Can you work these out from the model? Positions are in its coordinate system, mm. A direction names the side the tool comes from. Give positions to 0.01 mm unless a question says otherwise; leave off trailing zeros. Write each loop counter-clockwise with the first axis right and the second up, starting at its lowest first coordinate (ties: lowest second). Pieces come first, ordered by that corner, then holes. Notation, with made-up numbers: (68, 13.5) - (96, 13.5) arc R17 cw to (96, 21.5) - close; hole circle Ø4 at (-23.75, 30.25). An arc over 180 degrees is marked (long way). Use a Markdown table: item, result. Add a question column.
Autodesk Fusion 360 part; units mm, degrees
sketch "Sketch1" plane through (0, 0, 0) normal (0, 0, 1) x (1, 0, 0)
  line L0 (0, 0) -> (35, 0)
  line L1 (35, 30) -> (0, 30)
  line L2 (0, 30) -> (0, 0)
  circle A0 centre (35, 15) radius 2.25
  arc A1 (35, 0) -> (35, 30) centre (35, 15) ccw
  line L3 (15, 0) -> (15, 30)
  line L4 (15, 15) -> (0, 30) construction
  line L5 (7.5, 22.5) -> (7.5, 30) construction
  line L6 (7.5, 22.5) -> (0, 22.5) construction
  circle A2 centre (6.5, 23.5) radius 1
  circle A3 centre (8.5, 23.5) radius 1 construction
  circle A4 centre (8.5, 6.5) radius 1
  line L7 (15, 0) -> (0, 15) construction
  line L8 (7.5, 7.5) -> (7.5, 0) construction
  line L9 (7.5, 7.5) -> (15, 7.5) construction
  point P0 (40, 0)
  point P1 (15, 15)
  dimension "d1" = 30
  dimension "d7" = 35
  dimension "d8" = 35
  dimension "d9" = 4.5
  dimension "d14" = 2
  dimension "d36" = 2
extrude "Extrude1" add sketch "Sketch1" along normal blind 5 contours L0 L1 L2 L3 | L0 L1 A1 L3 | A0 | A2 | A4 makes body 1
hole "Hole1" at (8.5, 6.5, 0) at (6.5, 23.5, 0) direction (0, 0, 1) diameter 2 end through all counterbore diameter 2.3 counterbore depth 1 bodies 1 1
sketch "Sketch2" plane through (0, 0, 5) normal (0, 0, 1) x (-1, 0, 0)
  circle A0 centre (-8.5, -6.5) radius 1
  circle A1 centre (-6.5, -23.5) radius 1
  arc A2 (-35, 0) -> (-35, -30) centre (-35, -15) ccw
  line L0 (-35, -30) -> (0, -30)
  line L1 (0, -30) -> (0, 0)
  line L2 (0, 0) -> (-35, 0)
  circle A3 centre (-35, -15) radius 2.25
fillet "Fillet1" radius 2 3 edges at (17.5, 0, 0) (50, 15, 0) (17.5, 30, 0) on bodies 1
ref_plane "WorkPlane1" through (25, 15, 22.5) normal (0, 0, 1) x (1, 0, 0)
mirror "Mirror1" about plane through (25, 15, 22.5) normal (0, 0, 1) of bodies 1 makes body 2
extrude "Extrude2" cut sketch "Sketch2" against normal blind 4 contours A3 bodies 1
sketch "Sketch3" plane through (0, 0, 40) normal (0, 0, -1) x (1, 0, 0)
  circle A0 centre (8.5, -6.5) radius 1
  circle A1 centre (6.5, -23.5) radius 1
  arc A2 (35, -30) -> (35, 0) centre (35, -15) ccw
  line L0 (35, 0) -> (0, 0)
  line L1 (0, 0) -> (0, -30)
  line L2 (0, -30) -> (35, -30)
  line L3 (31.4, -14.9863) -> (24.6174, -26.7346)
  line L4 (35, -15) -> (24.8695, -28.0239) construction
  arc A3 (24.6174, -26.7346) -> (26.1812, -27.951) centre (25.4835, -27.2346) ccw
  line L5 (35.8992, -18.4859) -> (26.1812, -27.951)
  line L6 (31.4, -14.9863) -> (35.8992, -18.4859) construction
  arc A4 (35.8992, -18.4859) -> (31.4, -14.9863) centre (35, -15) ccw
  point P0 (35, -15)
  point P1 (35, -15)
  dimension "d30" = 2
  dimension "d31" = 5.7
  dimension "d32" = 16.5
  dimension "d33" = 7.2
extrude "Extrude3" cut sketch "Sketch3" against normal blind 1.5 contours L3 A3 L5 A4 bodies 2
hidden bodies 1
equation "d1 = breadth"
equation "breadth = 30 mm"
equation "length = 50 mm"
equation "d7 = length - d6"
equation "d8 = d7"
equation "d27 = ( 35 / 2 ) * 1 mm"
equation "d36 = d14"
Q1. If I drill on probe 1 along X at (y, z) = (23.5, 41.25); probe 2 along X at (y, z) = (3, 41.7); probe 3 along Y at (x, z) = (8.5, 42.4), over which ranges is the centre line in solid material (lowest first)? Write a range as [from, to].
Q2. Suppose I cut it at B-B (z = 42.05). Please give me the cut outline in (x, y).
Q3. Suppose I cut it at A-A (x = 6.5). Please give me the cut outline in (y, z).
Q4. If we mould it in two halves opening along Y, with no side actions, what happens to faces 4 (the cylindrical face through (17.74, 0.6, 44.43)), 5 (the flat face through (0, 15, 43)), 6 (the cylindrical face through (37.3, 12.23, 40.74))? For each: released by +Y, released by -Y, zero draft, split by the parting line, or undercut.
Q5. On a 3-axis mill with a long thin cutter (end or side, diameter ignored), from which of +Z, -Z, +X, -X, +Y, -Y can I reach the whole of each face in a straight line? I mean faces 1 (the flat face through (17, 30, 42)), 2 (the flat face through (28.056, 20.778, 40.74)), 3 (the cylindrical face through (7.8, 5.59, 44.49)). Say none if no direction works.
Derived:
| question | item | result |
|---|---|---|
| 1 | probe 1 | [0, 5.5], [7.5, 26.48], [30.75, 47.36] |
| 1 | probe 2 | [0, 44] |
| 1 | probe 3 | [0, 5.5], [7.5, 30] |
| 2 | outline | (0, 0) - (35, 0) arc R15 ccw to (35, 30) - (0, 30) - close; hole circle Ø2 at (6.5, 23.5); hole circle Ø2 at (8.5, 6.5) |
| 3 | outline | (0, 40) - (22.5, 40) - (22.5, 44) - (22.35, 44) - (22.35, 45) - (2, 45) arc R2 ccw to (0, 43) - close; (24.5, 40) - (30, 40) - (30, 43) arc R2 ccw to (28, 45) - (24.65, 45) - (24.65, 44) - (24.5, 44) - close |
| 4 | face 4 | released by -Y |
| 4 | face 5 | zero draft |
| 4 | face 6 | undercut |
| 5 | face 1 | +Z, -Z, +X, -X, +Y |
| 5 | face 2 | -Z |
| 5 | face 3 | +Z |
